Read the model definition and answer for the solid it produces. Units are mm, in the model's axes. Coordinates: 2 decimals unless noted, no trailing zeros. Loops run counter-clockwise (first coordinate to the right, second up) from the corner with the lowest first, then second, coordinate; pieces in that order, holes last. Notation, with made-up numbers: (3.5, 13) -> (28.5, 13) arc R13 cw to (28.5, 33) -> close; hole circle Ø10 at (62, -15). An arc over 180 degrees is marked (long way). Answer as CSV lines item,"result".
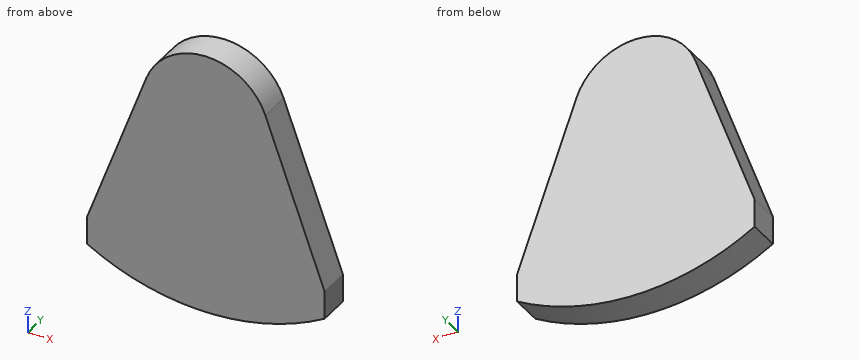
```python
from build123d import *

# Parameters (mm, degrees)
F2_DEPTH = 20


with BuildPart() as f2:
    # F1 (on Front) → F2 (new body)
    with BuildSketch(Plane.XZ):
        with BuildLine():
            ThreePointArc((37.5877048314, 128.680805733), (0, 155), (-37.5877048314, 128.680805733))
            Line((-37.5877048314, 128.680805733), (-75, 25.8913695474))
            Line((-75, 25.8913695474), (-75, 8.0961894323))
            ThreePointArc((-75, 8.0961894323), (0, -12), (75, 8.0961894323))
            Line((75, 8.0961894323), (75, 25.8913695474))
            Line((75, 25.8913695474), (37.5877048314, 128.680805733))
        make_face()
    extrude(amount=-F2_DEPTH)


solid = f2.part
```
Q1. Given pin 1 Ø12 at (x, y) = (41, 5.5) entering from -Z; pin 2 Ø1.5 at (x, y) = (30, 4) entering from +Z; pin 3 Ø8 at (y, z) = (14, 44.5) entering from -X, each flat-ended and moving along its own axis, determine where each tip first touches the part or whether it passes through.
Results:
pin 1,"stops at z = -7.86"
pin 2,"stops at z = 142.28"
pin 3,"stops at x = -69.68"
Q2. Find the intervals of material crossed by probe 1 along X at (y, z) = (6.25, 89); probe 2 along Z at (x, y) = (7, 10.5); probe 3 along Z at (x, y) = (22.5, 6), in increasing order. Write a range as [from, to].
Results:
probe 1,"x = [-52.03, 52.03]"
probe 2,"z = [-11.84, 154.38]"
probe 3,"z = [-10.3, 148.07]"
Q3. A cutting plane is placed at B-B, the plane x = 58.5. Write down the section's boundary in (y, z).
Results:
outline,"(0, -0.12) -> (20, -0.12) -> (20, 71.22) -> (0, 71.22) -> close"
Q4. A cutting plane is placed at C-C, the plane z = -1. Write down the section's boundary in (x, y).
Results:
outline,"(-56.38, 0) -> (56.38, 0) -> (56.38, 20) -> (-56.38, 20) -> close"
Q5. A cutting plane is placed at A-A, the plane y = 12. Write down the section's boundary in (x, z), and give its area (3 significant figures).
Results:
outline,"(-75, 8.1) arc R150 ccw to (75, 8.1) -> (75, 25.89) -> (37.59, 128.68) arc R40 ccw to (-37.59, 128.68) -> (-75, 25.89) -> close"
area,"17,700 mm²"
